Read the model definition and answer for the solid it produces. Units are mm, in the model's axes. Round coordinates to 2 decimals unless told otherwise and drop trailing zeros. Write each loop counter-clockwise with the first axis right and the second up, starting at its lowest first coordinate (ties: lowest second). Pieces come first, ordered by that corner, then holes.
from build123d import *

# Parameters (mm, degrees)
SKETCH045_W     = 30
SKETCH045_H     = 50
SKETCH045_R     = 2
PAD020_DEPTH    = 7
FILLET019_R     = 5
CHAMFER032_SIZE = 1


with BuildPart() as part:
    # Sketch045 → Pad020 (new body)
    with BuildSketch(Plane.XY):
        Rectangle(SKETCH045_W, SKETCH045_H)
        with Locations((-10, 20)):
            Circle(SKETCH045_R, mode=Mode.SUBTRACT)
        with Locations((10, 20)):
            Circle(SKETCH045_R, mode=Mode.SUBTRACT)
        with Locations((10, -20)):
            Circle(SKETCH045_R, mode=Mode.SUBTRACT)
        with Locations((-10, -20)):
            Circle(SKETCH045_R, mode=Mode.SUBTRACT)
    extrude(amount=-PAD020_DEPTH)

    # Fillet019
    fillet019_edges = [part.edges().sort_by_distance(p)[0] for p in [
        (15, -25, -3.5),
        (-15, -25, -3.5),
        (-15, 25, -3.5),
        (15, 25, -3.5),
    ]]
    fillet(fillet019_edges, radius=FILLET019_R)

    # Chamfer032
    chamfer032_edges = [part.edges().sort_by_distance(p)[0] for p in [
        (-15, 0, 0),
        (-13.535534, -23.535534, 0),
        (-13.535534, 23.535534, 0),
        (0, -25, 0),
        (0, 25, 0),
        (13.535534, -23.535534, 0),
        (13.535534, 23.535534, 0),
        (15, 0, 0),
        (-12, 20, 0),
        (8, 20, 0),
        (8, -20, 0),
        (-12, -20, 0),
        (-15, 0, -7),
        (-13.535534, -23.535534, -7),
        (-13.535534, 23.535534, -7),
        (0, -25, -7),
        (0, 25, -7),
        (13.535534, -23.535534, -7),
        (13.535534, 23.535534, -7),
        (15, 0, -7),
        (-12, 20, -7),
        (8, 20, -7),
        (8, -20, -7),
        (-12, -20, -7),
    ]]
    chamfer(chamfer032_edges, length=CHAMFER032_SIZE)


with BuildPart() as part_1:
    # Body015 placement: moved
    add(part.part.moved(Location((0, 80, 230))))


solid = part_1.part
Q1. A flat-ended cylindrical pin translates along its axis: pin 1 Ø5 at (x, y) = (-10, 100) entering from -Z. Find the tip coordinate at first contact, or state that the pin passes through.
Verdict:
pin 1: stops at z = 223.5
Q2. Section A-A (z = 229.5) is taken. Determine the outline of the cut face in (x, y).
Verdict:
outline: (-14.5, 60) arc R4.5 ccw to (-10, 55.5) - (10, 55.5) arc R4.5 ccw to (14.5, 60) - (14.5, 100) arc R4.5 ccw to (10, 104.5) - (-10, 104.5) arc R4.5 ccw to (-14.5, 100) - close; hole circle Ø5 at (-10, 60); hole circle Ø5 at (-10, 100); hole circle Ø5 at (10, 60); hole circle Ø5 at (10, 100)
Q3. Determine the mould class of faces 1 (the flat face through (14.5, 80.3, 223.5)), 2 (the flat face through (0, 105, 227)), 3 (the cylindrical face through (10, 102, 227)) for opening direction X: pulls with the +X half, pulls with the -X half, needs draft (parallel to the pull), parting line crosses it, or undercut.
Verdict:
face 1: pulls with the +X half
face 2: needs draft
face 3: undercut
Q4. Section B-B (y = 61) is taken. State how many separate pieces and enclosed holes the cut face has, then the cut area to 3 significant figures.
Verdict:
separate pieces: 3
enclosed holes: 0
area: 155 mm2
Q5. Straight lines are drawn through the part: probe 1 along Y at (x, z) = (-10, 226.9); probe 2 along X at (y, z) = (100, 227.4); probe 3 along X at (y, z) = (59.5, 226.5). For each, find the intervals that lie inside material, in ascending order.
Verdict:
probe 1: y = 55 to 58, 62 to 98, 102 to 105
probe 2: x = -15 to -12, -8 to 8, 12 to 15
probe 3: x = -14.97 to -11.94, -8.06 to 8.06, 11.94 to 14.97
